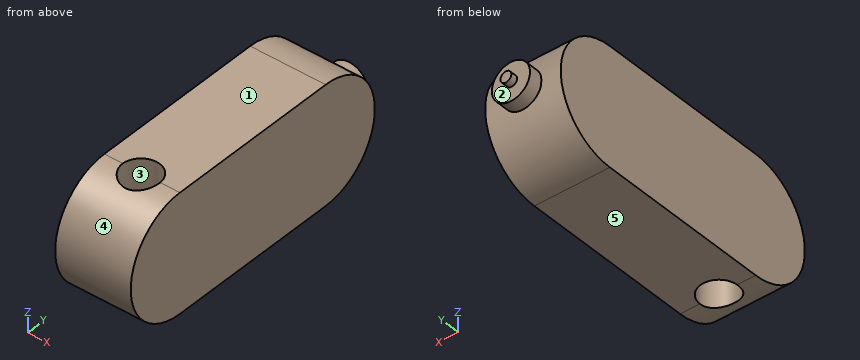
from build123d import *

# Parameters (mm, degrees)
BOSS_EXTRUDE2_DEPTH = 27
SKETCH6_R           = 6.674919097
CUT_EXTRUDE4_DEPTH  = 51
SKETCH7_R           = 6.817553131
BOSS_EXTRUDE3_DEPTH = 5
SKETCH8_R           = 1.936916623
BOSS_EXTRUDE4_DEPTH = 2.5


with BuildPart() as part:
    # Sketch3 → Boss-Extrude2 (new body)
    with BuildSketch(Plane(origin=(0, 0, 0), x_dir=(0, 0, -1), z_dir=(1, 0, 0))):
        with BuildLine():
            Line((-21.129473144, -21.663550217), (-21.129473144, 41.000059198))
            ThreePointArc((-21.129473144, 41.000059198), (0, 62.129532342), (21.129473144, 41.000059198))
            Line((21.129473144, 41.000059198), (21.129473144, -21.663550217))
            ThreePointArc((21.129473144, -21.663550217), (0, -42.793023362), (-21.129473144, -21.663550217))
        make_face()
    extrude(amount=BOSS_EXTRUDE2_DEPTH)

    # Sketch6 → Cut-Extrude4 (cut)
    with BuildSketch(Plane.XY.offset(22)):
        with Locations(Location((13.273045942, -21.878359575, 0), (0, 0, 1.844186398))):
            Circle(SKETCH6_R)
    extrude(amount=-CUT_EXTRUDE4_DEPTH, mode=Mode.SUBTRACT)

    # Sketch7 → Boss-Extrude3 (add)
    with BuildSketch(Plane(origin=(0, 62, 0), x_dir=(1, 0, 0), z_dir=(0, 1, 0))):
        with Locations(Location((13.747053519, 0, 0), (0, 0, 159.961468388))):
            Circle(SKETCH7_R)
    extrude(amount=BOSS_EXTRUDE3_DEPTH)

    # Sketch8 → Boss-Extrude4 (add)
    with BuildSketch(Plane(origin=(0, 67, 0), x_dir=(1, 0, 0), z_dir=(0, 1, 0))):
        with Locations(Location((13.472827278, 0, 0), (0, 0, 270))):
            Circle(SKETCH8_R)
    extrude(amount=BOSS_EXTRUDE4_DEPTH)


solid = part.part
The listing builds one solid part. Answer for the finished solid, in the listing's coordinates (mm). Face numbers are marked on the shaded views. A direction names the side the tool comes from. Give positions to 0.01 mm unless a question says otherwise; leave off trailing zeros. Write each loop counter-clockwise with the first axis right and the second up, starting at its lowest first coordinate (ties: lowest second). Pieces come first, ordered by that corner, then holes.
1) Given P1, Ø3.5, axis at x = 13.5, z = -3.5, coming from the -Y side; P2, Ø5, axis at x = 7, z = 0, coming from the -Y side; P3, Ø2, axis at x = 11.5, z = 3.5, coming from the -Y side, each flat-ended and moving along its own axis, determine where each tip first touches the part or whether it passes through.
2) Section A-A (z = -5.5) is taken. Write down the section's boundary in (x, y).
3) Section C-C (z = -0.5) is taken. Write down the section's boundary in (x, y).
4) A tool of negligible diameter and unlimited length cuts with its end or side. For the marked faces 1 and 2, from which of +Z, -Z, +X, -X, +Y, -Y can it reach the whole face along a straight path? Write none if from no direction.
5) Section D-D (x = 22.75) is taken. Write down the section's boundary in (y, z), and give its area (3 significant figures).
6) Find the intervals of material crossed by L1, parallel to Y at x = 15, z = -6.5; L2, parallel to Y at x = 14.25, z = 9.5; L3, parallel to Y at x = 19, z = -9, in increasing order.
7) For a pull along Y with two mould halves and no side action, classify the marked faces 3, 4 and 5 as pulls with the +Y half, pulls with the -Y half, needs draft (parallel to the pull), parting line crosses it, or undercut.
8) Section B-B (y = -25) is taken. Write down the section's boundary in (x, z), and give its area (3 significant figures).
Response:
1. P1: stops at y = -42.72
1. P2: stops at y = -42.79
1. P3: stops at y = -42.64
2. outline: (0, -42.06) - (27, -42.06) - (27, 61.4) - (0, 61.4) - close; (9.72, 62) - (17.78, 62) - (17.78, 67) - (9.72, 67) - close; hole circle Ø13.35 at (13.27, -21.88)
3. outline: (0, -42.79) - (27, -42.79) - (27, 62.12) - (20.55, 62.12) - (20.55, 67) - (15.34, 67) - (15.34, 69.5) - (11.6, 69.5) - (11.6, 67) - (6.95, 67) - (6.95, 62.12) - (0, 62.12) - close; hole circle Ø13.35 at (13.27, -21.88)
4. face 1: +Z, +X, -X, +Y, -Y
4. face 2: +Y
5. outline: (-21.66, -21.13) - (41, -21.13) arc R21.13 ccw to (41, 21.13) - (-21.66, 21.13) arc R21.13 ccw to start
5. area: 4,050 mm2
6. L1: y = -41.77 to -28.33, -15.43 to 61.1, 62 to 67
6. L2: y = -40.54 to -28.48, -15.28 to 59.87
6. L3: y = -40.78 to -25.31, -18.45 to 60.12
7. face 3: undercut
7. face 4: pulls with the -Y half
7. face 5: needs draft
8. outline: (0, -20.86) - (7.37, -20.86) - (7.37, 20.86) - (0, 20.86) - close; (19.17, -20.86) - (27, -20.86) - (27, 20.86) - (19.17, 20.86) - close
8. area: 634 mm2
